```python
from build123d import *

# Parameters (mm, degrees)
BOSS_EXTRUDE1_DEPTH = 3.5
SKETCH2_OUTSIDE_W   = 51.722
SKETCH2_OUTSIDE_H   = 49.042
SKETCH2_OUTSIDE_R   = 8.660254038
CUT_EXTRUDE1_DEPTH  = 7
CUT_EXTRUDE1_TAPER  = 60
SKETCH3_R           = 3
CUT_EXTRUDE2_DEPTH  = 8


with BuildPart() as part:
    # Sketch1 → Boss-Extrude1 (new body, symmetric)
    with BuildSketch(Plane(origin=(0, 0, 0), x_dir=(1, 0, 0), z_dir=(0, 1, 0))):
        Polygon((-10, 0), (-5, -8.660254038), (5, -8.660254038), (10, 0), (5, 8.660254038), (-5, 8.660254038), align=None)
    extrude(amount=BOSS_EXTRUDE1_DEPTH, both=True)

    # Sketch2 outside → Cut-Extrude1 (cut)
    with BuildSketch(Plane(origin=(0, 3.5, 0), x_dir=(1, 0, 0), z_dir=(0, 1, 0))):
        Rectangle(SKETCH2_OUTSIDE_W, SKETCH2_OUTSIDE_H)
        Circle(SKETCH2_OUTSIDE_R, mode=Mode.SUBTRACT)
    cut_extrude1 = extrude(amount=-CUT_EXTRUDE1_DEPTH, taper=CUT_EXTRUDE1_TAPER, mode=Mode.SUBTRACT)

    # Mirror1: Cut-Extrude1 across plane
    add(cut_extrude1.mirror(Plane.ZX), mode=Mode.SUBTRACT)

    # Sketch3 → Cut-Extrude2 (cut, through all)
    with BuildSketch(Plane(origin=(0, 3.5, 0), x_dir=(1, 0, 0), z_dir=(0, 1, 0))):
        Circle(SKETCH3_R)
    extrude(amount=-CUT_EXTRUDE2_DEPTH, mode=Mode.SUBTRACT)


solid = part.part
```
Geometry: final body of the model. Coordinates: model frame, mm. Round coordinates to 2 decimals unless told otherwise and drop trailing zeros. Order: outer loops, then holes, each group sorted by start corner. A loop starts at its lowest first (then second) coordinate and runs counter-clockwise, first axis right, second up. Notation, with made-up numbers: (26.5, 34) -> (51.5, 34) arc R15 cw to (51.5, 56) -> close; hole circle Ø4 at (-26.5, -16). An arc over 180 degrees is marked (long way). Use one line per item in the form item = value.
(1) Draft query along Z for faces 1 (the face through (4.5, -3.3, 7.8)), 2 (the face through (4.5, 3.3, -7.8)), 3 (the face through (-3, 0, 0)), 4 (the face through (-8.99, 3.31, 0.02)). Return one class per face: pulls with the +Z half, pulls with the -Z half, needs draft (parallel to the pull), parting line crosses it, or undercut.
Results list:
face_1 = pulls with the +Z half
face_2 = pulls with the -Z half
face_3 = undercut
face_4 = parting line crosses it
(2) Section A-A on y = 1.25. Return loops of the section in (x, z).
Results list:
outline = (-10, 0) -> (-5, -8.66) -> (5, -8.66) -> (10, 0) -> (5, 8.66) -> (-5, 8.66) -> close; hole circle Ø6 at (0, 0)
(3) Ray query, probe 1 along X at (y, z) = (-3, -0.75); probe 2 along X at (y, z) = (3.25, 0.5); probe 3 along Z at (x, y) = (-1.75, -2). Return the intervals inside material, ascending. Write a range as [from, to].
Results list:
probe_1 = [-9.5, -2.9], [2.9, 9.5]
probe_2 = [-9.08, -2.96], [2.96, 9.08]
probe_3 = [-8.66, -2.44], [2.44, 8.66]
(4) First-contact query: pin 1 Ø3 at (y, z) = (-1, 0.5) entering from -X; pin 2 Ø4 at (y, z) = (0.5, 4) entering from +X. Flat tips, straight axial feed; report the tip coordinate or a pass-through.
Results list:
pin_1 = -10
pin_2 = 8.85
